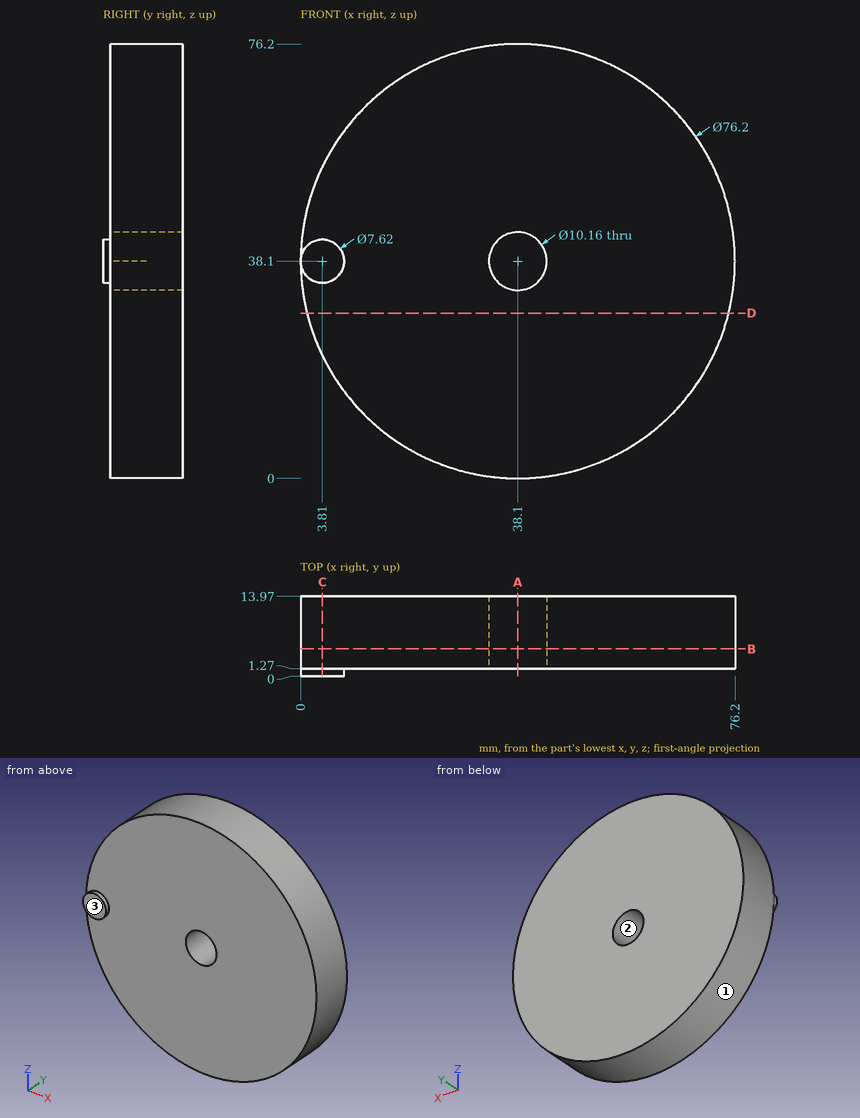
Answer from the drawing. Dimensions are ordinates in mm from the lowest x, y and z of the part. Round coordinates to 2 decimals unless told otherwise and drop trailing zeros. Write each loop counter-clockwise with the first axis right and the second up, starting at its lowest first coordinate (ties: lowest second). Pieces come first, ordered by that corner, then holes. Notation, with made-up numbers: M 51,-15 L 70,-15 A22 ccw 70,24 Z; hole C 41.25,-29 d4. An arc over 180 degrees is marked long. Write each question's results on one line, items separated by ' | '. Start each with the question number.
Item 1: Find section D-D on z = 29. Write down the section's boundary in (x, y).
Item 2: The mould has two halves that part along X. Classify the marked faces 1, 2 and 3: +X half, -X half, draft (parallel to the pull), parting line (faces both ways), or undercut.
Item 3: Find section C-C on x = 3.81. Write down the section's boundary in (y, z), and give its area (3 significant figures).
Item 4: Find section B-B on y = 4.75. Write down the section's boundary in (x, z), and give its area (3 significant figures).
Item 5: Given pin 1 Ø8 at (x, z) = (38.1, 38.1) entering from +Y; pin 2 Ø2 at (y, z) = (9.5, 50) entering from +X; pin 3 Ø2 at (x, y) = (28.5, 5) entering from -Z; pin 4 Ø1 at (x, z) = (22.5, 8.5) entering from -Y, each flat-ended and moving along its own axis, determine where each tip first touches the part or whether it passes through.
Item 6: Find section A-A on x = 38.1. Write down the section's boundary in (y, z), and give its area (3 significant figures).
Item 7: Straight lines are drawn through the part: probe 1 along Z at (x, y) = (38.1, 10.5); probe 2 along Y at (x, z) = (29, 56.5); probe 3 along Z at (x, y) = (72, 11.5). For each, find the intervals that lie inside material, in ascending order.
Answer block:
1) outline: M 1.1,1.27 L 75.1,1.27 L 75.1,13.97 L 1.1,13.97 Z
2) face 1: parting line | face 2: undercut | face 3: draft
3) outline: M 0,34.29 L 1.27,34.29 L 1.27,21.49 L 13.97,21.49 L 13.97,54.71 L 1.27,54.71 L 1.27,41.91 L 0,41.91 Z | area: 432 mm²
4) outline: C 38.1,38.1 d76.2; hole C 38.1,38.1 d10.16 | area: 4,480 mm²
5) pin 1: passes through | pin 2: stops at x = 74.61 | pin 3: stops at z = 0.98 | pin 4: stops at y = 1.27
6) outline: M 1.27,0 L 13.97,0 L 13.97,33.02 L 1.27,33.02 Z; M 1.27,43.18 L 13.97,43.18 L 13.97,76.2 L 1.27,76.2 Z | area: 839 mm²
7) probe 1: z = 0 to 33.02, 43.18 to 76.2 | probe 2: y = 1.27 to 13.97 | probe 3: z = 20.71 to 55.49
